Source: CAD feature listing. Evaluate the final solid. Frame: model axes, mm. Give positions to 0.01 mm unless a question says otherwise; leave off trailing zeros. Order: outer loops, then holes, each group sorted by start corner. A loop starts at its lowest first (then second) coordinate and runs counter-clockwise, first axis right, second up.
```python
from build123d import *

# Parameters (mm, degrees)
SKETCH1_W                = 33.8
SKETCH1_H                = 37.5
BOSS_EXTRUDE_NOANT_DEPTH = 1
SKETCH2_W                = 41.9
SKETCH2_H                = 37.5
BOSS_EXTRUDE_ANT_DEPTH   = 1
SKETCH3_R                = 1.25
HOLES_DEPTH              = 46.914839649
CORNERS_DEPTH            = 46.914839649
SKETCH5_W                = 13
SKETCH5_H                = 5.65
CUT_EXTRUDE1_DEPTH       = 46.914839649
SKETCH6_W                = 7.8
SKETCH6_H                = 5.2
CUT_EXTRUDE2_DEPTH       = 46.914839649


with BuildPart() as part:
    # Sketch1 → Boss-Extrude-NoAnt (new body)
    with BuildSketch(Plane.XY):
        with Locations((-16.9, 0)):
            Rectangle(SKETCH1_W, SKETCH1_H)
    extrude(amount=BOSS_EXTRUDE_NOANT_DEPTH)

    # Sketch2 → Boss-Extrude-Ant (add)
    with BuildSketch(Plane.XY):
        with Locations((20.95, 0)):
            Rectangle(SKETCH2_W, SKETCH2_H)
    extrude(amount=BOSS_EXTRUDE_ANT_DEPTH)

    # Sketch3 → Holes (cut, through all)
    with BuildSketch(Plane(origin=(0, 0, 0), x_dir=(-1, 0, 0), z_dir=(0, 0, -1))):
        with Locations((31.45, -16.4)):
            Circle(SKETCH3_R)
        with Locations((-39.55, -16.4)):
            Circle(SKETCH3_R)
        with Locations((-39.55, 16.4)):
            Circle(SKETCH3_R)
        with Locations((31.45, 16.4)):
            Circle(SKETCH3_R)
    extrude(amount=-HOLES_DEPTH, mode=Mode.SUBTRACT)

    # Sketch4 → Corners (cut, through all)
    with BuildSketch(Plane(origin=(0, 0, 0), x_dir=(-1, 0, 0), z_dir=(0, 0, -1))):
        Polygon((-41.9, 18.75), (-40.5, 18.75), (-41.9, 17.35), align=None)
        Polygon((-41.9, -17.35), (-41.9, -18.75), (-40.5, -18.75), align=None)
        Polygon((33.8, -18.75), (32.4, -18.75), (33.8, -17.35), align=None)
        Polygon((33.8, 17.35), (33.8, 18.75), (32.4, 18.75), align=None)
    extrude(amount=-CORNERS_DEPTH, mode=Mode.SUBTRACT)

    # Sketch5 → Cut-Extrude1 (cut, through all)
    with BuildSketch(Plane.XY.offset(1)):
        with Locations((-15, -15.925)):
            Rectangle(SKETCH5_W, SKETCH5_H)
    extrude(amount=-CUT_EXTRUDE1_DEPTH, mode=Mode.SUBTRACT)

    # Sketch6 → Cut-Extrude2 (cut, through all)
    with BuildSketch(Plane(origin=(0, 0, 0), x_dir=(-1, 0, 0), z_dir=(0, 0, -1))):
        with Locations((22.65, 16.15)):
            Rectangle(SKETCH6_W, SKETCH6_H)
    extrude(amount=-CUT_EXTRUDE2_DEPTH, mode=Mode.SUBTRACT)


solid = part.part
```
1) Pin query (flat end, axial travel): pin 1 (0.5 mm diameter, centred on x = -14, z = 0.5, fed in from -Y). Return the tip coordinate at first contact, or that it passes through.
Report:
pin 1: stops at y = -13.1
2) Section query A-A, the plane y = -16.4. Return the cut outline in (x, z), and give its area (3 significant figures).
Report:
outline: (-33.8, 0) - (-32.7, 0) - (-32.7, 1) - (-33.8, 1) - close; (-30.2, 0) - (-21.5, 0) - (-21.5, 1) - (-30.2, 1) - close; (-8.5, 0) - (38.3, 0) - (38.3, 1) - (-8.5, 1) - close; (40.8, 0) - (41.9, 0) - (41.9, 1) - (40.8, 1) - close
area: 57.7 mm2
3) Section query D-D, the plane y = 16.4. Return the cut outline in (x, z), and give its area (3 significant figures).
Report:
outline: (-33.8, 0) - (-32.7, 0) - (-32.7, 1) - (-33.8, 1) - close; (-30.2, 0) - (-26.55, 0) - (-26.55, 1) - (-30.2, 1) - close; (-18.75, 0) - (38.3, 0) - (38.3, 1) - (-18.75, 1) - close; (40.8, 0) - (41.9, 0) - (41.9, 1) - (40.8, 1) - close
area: 62.9 mm2
4) Section query C-C, the plane z = 0.7. Return the cut outline in (x, y), and give its area (3 significant figures).
Report:
outline: (-33.8, -17.35) - (-32.4, -18.75) - (-21.5, -18.75) - (-21.5, -13.1) - (-8.5, -13.1) - (-8.5, -18.75) - (40.5, -18.75) - (41.9, -17.35) - (41.9, 17.35) - (40.5, 18.75) - (-18.75, 18.75) - (-18.75, 13.55) - (-26.55, 13.55) - (-26.55, 18.75) - (-32.4, 18.75) - (-33.8, 17.35) - close; hole circle Ø2.5 at (-31.45, -16.4); hole circle Ø2.5 at (-31.45, 16.4); hole circle Ø2.5 at (39.55, -16.4); hole circle Ø2.5 at (39.55, 16.4)
area: 2,700 mm2
5) Draft query along X for faces 1 (the flat face through (41.19, 18.06, 0.49)), 2 (the cylindrical face through (-30.2, 16.45, 0.49)), 3 (the flat face through (-33.09, -18.06, 0.49)). Return one class per face: +X half, -X half, draft (parallel to the pull), parting line (faces both ways), or undercut.
Report:
face 1: +X half
face 2: undercut
face 3: -X half
6) Section query B-B, the plane x = 39.55. Return the cut outline in (y, z).
Report:
outline: (-18.75, 0) - (-17.65, 0) - (-17.65, 1) - (-18.75, 1) - close; (-15.15, 0) - (15.15, 0) - (15.15, 1) - (-15.15, 1) - close; (17.65, 0) - (18.75, 0) - (18.75, 1) - (17.65, 1) - close
7) Material intervals for L1, parallel to Y at x = 39.55, z = 0.65; L2, parallel to Y at x = -26.5, z = 0.75, sorted ascending.
Report:
L1: y = -18.75 to -17.65, -15.15 to 15.15, 17.65 to 18.75
L2: y = -18.75 to 13.55
